```python
from build123d import *

# Parameters (mm, degrees)
F0_R     = 63.5
F1_DEPTH = 127
F3_DEPTH = 76.2


with BuildPart() as f1:
    # F0 (on Front) → F1 (new body, symmetric)
    with BuildSketch(Plane.XZ):
        Circle(F0_R)
    extrude(amount=F1_DEPTH, both=True)

    # F2 (on face) → F3 (join)
    with BuildSketch(Plane.XZ.offset(127)):
        Polygon((87.400252, -63.5), (87.400252, 63.5), (-33.383926, 102.745158), (-108.032653, 0), (-33.383926, -102.745158), align=None)
    extrude(amount=F3_DEPTH)

    # F4 (on Top) → F5 (revolve, cut)
    with BuildSketch(Plane.XY):
        Polygon((178.573892, -101.46219), (66.709772, -211.132884), (178.573892, -339.390486), align=None)
    revolve(axis=Axis((0, -117.441341, 0), (0, -1, 0)), mode=Mode.SUBTRACT)


solid = f1.part
```
Can you work these out from the model? Positions are in its coordinate system, mm. A direction names the side the tool comes from. Coordinates: 2 decimals unless noted, no trailing zeros. Loops run counter-clockwise (first coordinate to the right, second up) from the corner with the lowest first, then second, coordinate; pieces in that order, holes last. Notation, with made-up numbers: (2.5, 0.5) -> (49.5, 0.5) arc R19 ccw to (49.5, 28.5) -> close; hole circle Ø4 at (5, -6). An arc over 180 degrees is marked (long way). Put each result on its own line as item: value. Start each with the question number.
Q1. I want a section at B-B (y = -100). Write out the boundary of the cut face in (x, z), plus the area to 3 significant figures.
Q2. If I drill on line 1 (Z direction, x = -1, y = -63); line 2 (X direction, y = -84, z = -14); line 3 (Z direction, x = 0.5, y = -156), over which ranges is the centre line in solid material (lowest first)? Write a range as [from, to].
Q3. I'm going to push flat-ended pins straight in: P1, Ø2, axis at x = 6, z = -69.5, coming from the +Y side; P2, Ø12, axis at y = -89, z = -17, coming from the +X side; P3, Ø12, axis at x = -64, z = 62, coming from the -Y side. Where does each tip first touch, or does it pass through?
Q4. I want a section at A-A (x = 0). Write out the boundary of the cut face in (y, z), plus the area to 3 significant figures.
Q5. For faces 1 (the face through (-76.34, -201.62, 3.36)), 2 (the face through (10, -127, -67)), which set-ups out of +Z, -Z, +X, -X, +Y, -Y let a thin tool reach every point of the face, with its end or its side?
Taken from the geometry:
1. outline: circle Ø127 at (0, 0)
1. area: 12,700 mm2
2. line 1: z = [-63.49, 63.49]
2. line 2: x = [-61.94, 61.94]
2. line 3: z = [-91.74, 91.74]
3. P1: stops at y = -127
3. P2: stops at x = 62.54
3. P3: stops at y = -195.06
4. outline: (-203.2, -74.8) -> (-186.44, -91.9) -> (-127, -91.9) -> (-127, -63.5) -> (127, -63.5) -> (127, 63.5) -> (-127, 63.5) -> (-127, 91.9) -> (-186.44, 91.9) -> (-203.2, 74.8) -> close
4. area: 46,000 mm2
5. face 1: -Y
5. face 2: +Y
